Solid Edge part; units mm, degrees
sketch "Sketch1" plane through (0, 0, 0) normal (0, 0, 1) x (1, 0, 0)
  circle A0 centre (0, 0) radius 12.5
  circle A1 centre (0, 0) radius 17.5
extrude "Protrusion1" add sketch "Sketch1" along normal blind 1.75
sketch "Sketch2" plane through (0, 0, 1.75) normal (0, 0, 1) x (1, 0, 0)
  circle A0 centre (0, 15) radius 1
  circle A1 centre (15, 0) radius 1
  circle A2 centre (0, -15) radius 1
  circle A3 centre (-15, 0) radius 1
extrude "VaciadoExtruido_1" cut sketch "Sketch2" against normal blind 0.25
sketch "Sketch3" plane through (0, 0, 0) normal (0, 0, -1) x (0, 1, 0)
  line L0 (1.8274, 13.8802) -> (2.0884, 15.8631)
  line L1 (-1.8274, 13.8802) -> (-2.0884, 15.8631)
  arc A0 (-1.8274, 13.8802) -> (1.8274, 13.8802) centre (0, 0) cw
  arc A1 (-2.0884, 15.8631) -> (2.0884, 15.8631) centre (0, 0) cw
extrude "ProtrusiónExtruida_2" add sketch "Sketch3" along normal blind 0.1
pattern_circular "Pattern1" count 8 over 360 about axis through (0, 0, 0) along (0, 0, 1) of "ProtrusiónExtruida_2"
sketch "Sketch4" plane through (0, 0, 1.75) normal (0, 0, 1) x (0, 1, 0)
  line L0 (6.6565, -13.2417) -> (4.6565, -14.0701)
  line L1 (4.6565, -14.0701) -> (5.0707, -15.0701)
  line L2 (7.0707, -14.2417) -> (5.0707, -15.0701)
  line L3 (6.6565, -13.2417) -> (7.0707, -14.2417)
extrude "ProtrusiónExtruida_3" add sketch "Sketch4" along normal blind 1
pattern_circular "Pattern3" count 8 over 360 about axis through (0, 0, 1.75) along (0, 0, 1) of "ProtrusiónExtruida_3"
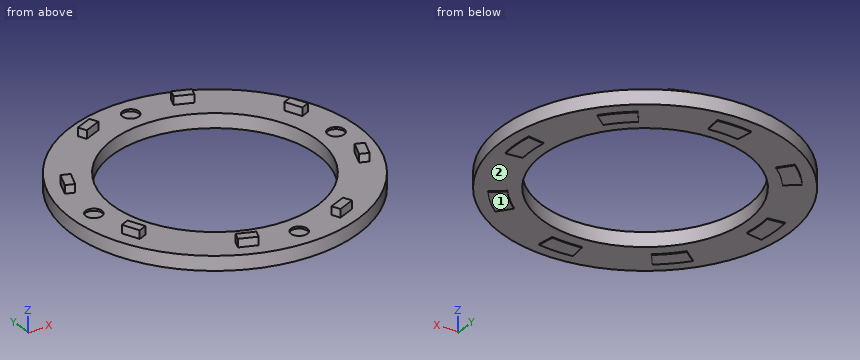
The model under review builds one solid part; all positions refer to its coordinate system, in mm. Face numbers are marked on the shaded views. Give positions to 0.01 mm unless a question says otherwise; leave off trailing zeros. Loops run counter-clockwise (first coordinate to the right, second up) from the corner with the lowest first, then second, coordinate; pieces in that order, holes last. Notation, with made-up numbers: (-31, 33) -> (-7, 33) arc R13 cw to (-7, 45) -> close; hole circle Ø2 at (14, 21.5). An arc over 180 degrees is marked (long way). Answer as a JSON object with one key per item and string values. Group by question number.
Q1. Take a section at A-A (y = 0). Write out the cut boundary in (x, z), plus the area to 3 significant figures.
Q2. Draft analysis for pull direction X (two halves, no side actions). For the marked faces 1 and 2, state which applies: pulls with the +X half, pulls with the -X half, needs draft (parallel to the pull), parting line crosses it, or undercut.
Q3. Wall thickness on line 1 along Y through (x, z) = (0, 1.6); line 2 along Y through (x, z) = (0, 1.3); line 3 along Y through (x, z) = (-10, 1): over which ranges is each line inside the solid? List them lowest first.
Q4. Take a section at D-D (x = 4). Write out the cut boundary in (y, z), plus the area to 3 significant figures.
Q5. Take a section at C-C (z = 0.75). Write out the cut boundary in (x, y), plus the area to 3 significant figures.
Q6. Insertion check: pin 1 (2 mm diameter, centred on x = 15, y = 0.5, fed in from +Z); pin 2 (1.5 mm diameter, centred on x = 6.5, z = 1, fed in from -Y); pin 3 (8 mm diameter, centred on x = 0, y = -12, fed in from -Z); pin 4 (1 mm diameter, centred on x = 0, y = 15, fed in from +Z). Each pin has a flat end and moves straight along its axis. Give the tip position at first contact, or say it passes through.
Answer below:
{
 "1": {"outline": "(-17.5, 0) -> (-16, 0) -> (-16, -0.1) -> (-14, -0.1) -> (-14, 0) -> (-12.5, 0) -> (-12.5, 1.75) -> (-14, 1.75) -> (-14, 1.5) -> (-16, 1.5) -> (-16, 1.75) -> (-17.5, 1.75) -> close; (12.5, 0) -> (14, 0) -> (14, -0.1) -> (16, -0.1) -> (16, 0) -> (17.5, 0) -> (17.5, 1.75) -> (16, 1.75) -> (16, 1.5) -> (14, 1.5) -> (14, 1.75) -> (12.5, 1.75) -> close", "area": "16.9 mm2"},
 "2": {"face 1": "needs draft", "face 2": "undercut"},
 "3": {"line 1": "y = -17.5 to -16, -14 to -12.5, 12.5 to 14, 16 to 17.5", "line 2": "y = -17.5 to -12.5, 12.5 to 17.5", "line 3": "y = -14.36 to -7.5, 7.5 to 14.36"},
 "4": {"outline": "(-17.04, 0) -> (-11.84, 0) -> (-11.84, 1.75) -> (-17.04, 1.75) -> close; (11.84, 0) -> (17.04, 0) -> (17.04, 1.75) -> (11.84, 1.75) -> close", "area": "18.2 mm2"},
 "5": {"outline": "circle Ø35 at (0, 0); hole circle Ø25 at (0, 0)", "area": "471 mm2"},
 "6": {"pin 1": "stops at z = 1.75", "pin 2": "stops at y = -16.53", "pin 3": "stops at z = -0.1", "pin 4": "stops at z = 1.5"}
}
